Autodesk Inventor part; units mm, degrees
ref_plane "YZ Plane" through (0, 0, 0) normal (1, 0, 0) x (0, 1, 0)
ref_plane "XZ Plane" through (0, 0, 0) normal (0, 1, 0) x (-1, 0, 0)
ref_plane "XY Plane" through (0, 0, 0) normal (0, 0, 1) x (1, 0, 0)
sketch "Sketch1" plane through (0, 0, 0) normal (0, 1, 0) x (-1, 0, 0)
  line L0 (0, 0) -> (-20, 0)
  line L1 (-20, 0) -> (-20, -80)
  line L2 (-20, -80) -> (0, -80)
  line L3 (0, -80) -> (0, 0)
  line L4 (-10, 0) -> (-10, -10)
  line L5 (-10, -10) -> (-10, -70) construction
  line L6 (-12.75, -10) -> (-12.75, -70)
  line L7 (-7.25, -70) -> (-7.25, -10)
  arc A0 (-7.25, -10) -> (-12.75, -10) centre (-10, -10) ccw
  arc A1 (-12.75, -70) -> (-7.25, -70) centre (-10, -70) ccw
  line L8 (-10, -10) -> (50, -10) construction
  point P0 (-10, -40)
  dimension "d0" = 20
  dimension "d1" = 80
  dimension "d2" = 10
  dimension "d3" = 60
  dimension "d4" = 90
  dimension "d5" = 5.5
extrude "Extrusion1" add sketch "Sketch1" along normal blind 3
fillet "Fillet1" radius 5 4 edges at (20, 1.5, 0) (0, 1.5, 0) (20, 1.5, -80) (0, 1.5, -80)
properties part number "Carriage_Horizontal_Spacer"
Work out the finished part from the listing and answer in its coordinate system (mm). A direction names the side the tool comes from. Round coordinates to 2 decimals unless told otherwise and drop trailing zeros. Write each loop counter-clockwise with the first axis right and the second up, starting at its lowest first coordinate (ties: lowest second). Pieces come first, ordered by that corner, then holes. Notation, with made-up numbers: (16.5, 37.25) -> (67.5, 37.25) arc R5 ccw to (67.5, 46.25) -> close; hole circle Ø6 at (84, 79). An arc over 180 degrees is marked (long way). Answer as CSV lines item,"result". Start each with the question number.
(1) Find the intervals of material crossed by probe 1 along X at (y, z) = (0.95, -30); probe 2 along Z at (x, y) = (11, 0.5); probe 3 along Z at (x, y) = (12, 2.4), in increasing order.
(2) The part is cut by section D-D, the plane x = 18. Give the vertices of the cut face in (y, z), then the cut area to 3 significant figures.
(3) The part is cut by section B-B, the plane x = 10. Give the vertices of the cut face in (y, z).
(4) The part is cut by section C-C, the plane y = 2.05. Give the vertices of the cut face in (x, z).
(5) The part is cut by section A-A, the plane z = -26. Give the vertices of the cut face in (x, y).
(6) A tool of negligible diameter and unlimited length cuts with its end or side. For faces 1 (the flat face through (20, 1, -40)), 2 (the cylindrical face through (9.94, 1.48, -72.75)), from which of +Z, -Z, +X, -X, +Y, -Y can it reach the whole face along a straight path? Write none if from no direction.
(7) The mould has two halves that part along X. Classify faces 3 (the cylindrical face through (19, 2, -78)), 4 (the cylindrical face through (1, 2, -2)), 5 (the flat face through (10, 1, -80)), 6 (the flat face through (7.25, 1, -40)): +X half, -X half, draft (parallel to the pull), parting line (faces both ways), or undercut.
Output values:
1,probe 1,"x = 0 to 7.25, 12.75 to 20"
1,probe 2,"z = -80 to -72.56, -7.44 to 0"
1,probe 3,"z = -80 to -71.89, -8.11 to 0"
2,outline,"(0, -79) -> (3, -79) -> (3, -1) -> (0, -1) -> close"
2,area,"234 mm²"
3,outline,"(0, -80) -> (3, -80) -> (3, -72.75) -> (0, -72.75) -> close; (0, -7.25) -> (3, -7.25) -> (3, 0) -> (0, 0) -> close"
4,outline,"(0, -75) arc R5 ccw to (5, -80) -> (15, -80) arc R5 ccw to (20, -75) -> (20, -5) arc R5 ccw to (15, 0) -> (5, 0) arc R5 ccw to (0, -5) -> close; hole (7.25, -70) arc R2.75 ccw to (12.75, -70) -> (12.75, -10) arc R2.75 ccw to (7.25, -10) -> close"
5,outline,"(0, 0) -> (7.25, 0) -> (7.25, 3) -> (0, 3) -> close; (12.75, 0) -> (20, 0) -> (20, 3) -> (12.75, 3) -> close"
6,face 1,"+Z, -Z, +X, +Y, -Y"
6,face 2,"+Y, -Y"
7,face 3,"+X half"
7,face 4,"-X half"
7,face 5,"draft"
7,face 6,"undercut"
